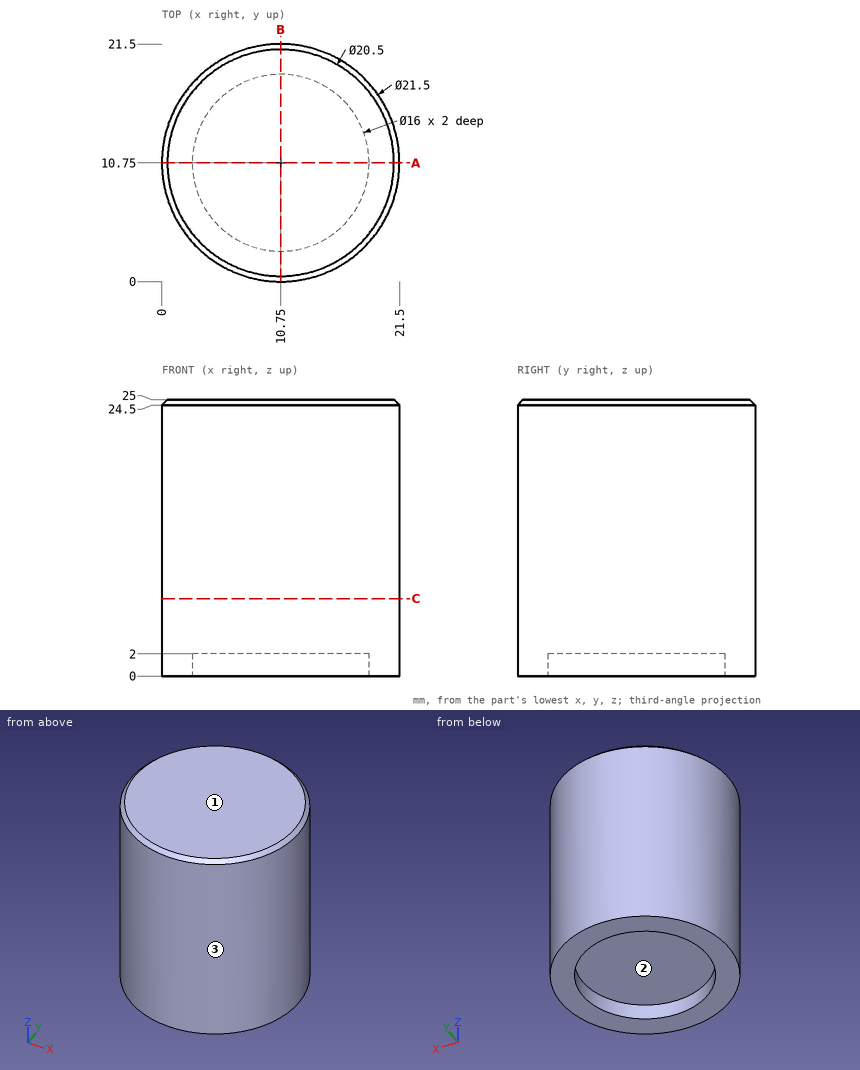
Study the drawing (mm; zero at the part's minimum x, y, z) and answer. Give positions to 0.01 mm unless a question says otherwise; leave off trailing zeros. Write each loop counter-clockwise with the first axis right and the second up, starting at its lowest first coordinate (ties: lowest second). Pieces come first, ordered by that corner, then holes. Notation, with made-up numbers: (58.5, 32) - (73.5, 32) arc R21 cw to (73.5, 65) - close; hole circle Ø8 at (56, 51.25). An arc over 180 degrees is marked (long way). Write item = value, one per line. Start each with the question number.
Item 1: Find section C-C (z = 7). Give the vertices of the cut face in (x, y), then the cut area to 3 significant figures.
Item 2: Find the intervals of material crossed by probe 1 along Y at (x, z) = (10.75, 1.35); probe 2 along Z at (x, y) = (18, 7.5); probe 3 along Y at (x, z) = (19.75, 5.75), in increasing order. Write a range as [from, to].
Item 3: The mould has two halves that part along X. Classify the marked faces 1, 2 and 3: +X half, -X half, draft (parallel to the pull), parting line (faces both ways), or undercut.
Item 4: Find section A-A (y = 10.75). Give the vertices of the cut face in (x, z).
Item 5: Each of these flat-tipped pins is pushed along its axis until it touches: P1, Ø1, axis at y = 3.5, z = 16, coming from the -X side; P2, Ø2, axis at y = 13, z = 22.5, coming from the +X side; P3, Ø4, axis at y = 4, z = 9, coming from the -X side. Where does it stop, or does it pass through?
Response:
q1.outline = circle Ø21.5 at (10.75, 10.75)
q1.area = 363 mm²
q2.probe_1 = [0, 2.75], [18.75, 21.5]
q2.probe_2 = [2, 25]
q2.probe_3 = [4.87, 16.63]
q3.face_1 = draft
q3.face_2 = undercut
q3.face_3 = parting line
q4.outline = (0, 0) - (2.75, 0) - (2.75, 2) - (18.75, 2) - (18.75, 0) - (21.5, 0) - (21.5, 24.5) - (21, 25) - (0.5, 25) - (0, 24.5) - close
q5.P1 = 2.38
q5.P2 = 21.43
q5.P3 = 1.11
